Autodesk Inventor part; units mm, degrees
ref_plane "YZ Plane" through (0, 0, 0) normal (1, 0, 0) x (0, 1, 0)
ref_plane "XZ Plane" through (0, 0, 0) normal (0, 1, 0) x (-1, 0, 0)
ref_plane "XY Plane" through (0, 0, 0) normal (0, 0, 1) x (1, 0, 0)
sketch "Sketch1" plane through (0, 0, 0) normal (0, 1, 0) x (-1, 0, 0)
  circle A0 centre (0, 0) radius 19.4
  line L0 (0, 0) -> (0, -10.9961) construction
  circle A1 centre (0, -45) radius 19.4
  circle A2 centre (45, 22.5) radius 19.4
  circle A3 centre (45, -22.5) radius 19.4
  circle A4 centre (45, -67.5) radius 19.4
  line L1 (-27.5, -92.5) -> (72.5, -92.5)
  line L2 (72.5, -92.5) -> (72.5, 47.5)
  line L3 (72.5, 47.5) -> (-27.5, 47.5)
  line L4 (-27.5, 47.5) -> (-27.5, -92.5)
  line L5 (-27.5, -92.5) -> (72.5, 47.5) construction
  line L6 (72.5, -92.5) -> (-27.5, 47.5) construction
  point P0 (22.5, -22.5)
  dimension "d0" = 38.8
  dimension "d3" = 45
  dimension "d8" = 38.8
  dimension "d9" = 45
  dimension "d10" = 22.5
  dimension "d13" = 45
  dimension "d18" = 22.5
  dimension "d19" = 50
  dimension "d20" = 70
  dimension "d21" = 22.5
extrude "Extrusion1" add sketch "Sketch1" along normal blind 10
extrude "Extrusion2" add sketch "Sketch1" against normal blind 3 contours A0 | A1 | A2 | A3 | A4 | L4 L3 L2 L1
sketch "Sketch3" plane through (0, 10, 0) normal (0, 1, 0) x (1, 0, 0)
  line L0 (24.5, 89.5) -> (19.5, 89.5)
  line L1 (19.5, 89.5) -> (19.5, 84.5)
  line L2 (19.5, 84.5) -> (24.5, 84.5)
  line L3 (24.5, 84.5) -> (24.5, 89.5)
  line L4 (24.5, -39.5) -> (19.5, -39.5)
  line L5 (19.5, -39.5) -> (19.5, -44.5)
  line L6 (19.5, -44.5) -> (24.5, -44.5)
  line L7 (24.5, -44.5) -> (24.5, -39.5)
  line L8 (-64.5, -44.5) -> (-69.5, -44.5)
  line L9 (-69.5, -44.5) -> (-69.5, -39.5)
  line L10 (-69.5, -39.5) -> (-64.5, -39.5)
  line L11 (-64.5, -39.5) -> (-64.5, -44.5)
  line L12 (-64.5, 89.5) -> (-69.5, 89.5)
  line L13 (-69.5, 89.5) -> (-69.5, 84.5)
  line L14 (-69.5, 84.5) -> (-64.5, 84.5)
  line L15 (-64.5, 84.5) -> (-64.5, 89.5)
  line L16 (27.5, -47.5) -> (27.5, 92.5)
  line L17 (27.5, 92.5) -> (-72.5, 92.5)
  line L18 (-72.5, -47.5) -> (27.5, -47.5)
  line L19 (-72.5, 92.5) -> (-72.5, -47.5)
  point P0 (0, 0)
  dimension "d26" = 5
  dimension "d27" = 3
  dimension "d28" = 3
  dimension "d29" = 5
  dimension "d30" = 3
  dimension "d31" = 3
  dimension "d32" = 5
  dimension "d33" = 3
  dimension "d34" = 5
extrude "Extrusion3" cut sketch "Sketch3" against normal blind 2 contours L3 L2 L1 L0 | L7 L6 L5 L4 | L8 L9 L10 L11 | L15 L14 L13 L12
equation "\"d0\" = bottleDiameter"
equation "\"d3\" = bottleDistance"
equation "\"d8\" = bottleDiameter"
equation "\"d13\" = bottleDistance"
equation "\"capDiameter\" = 29.5"
equation "\"bottleLen\" = 81.3"
equation "\"bottleDiameter\" = 38.8"
equation "\"tubeInsideDiameter\" = 2"
equation "\"tubeOutsideDiameter\" = 5.4"
equation "\"tick\" = 2"
equation "\"connectorDiameter\" = 35"
equation "\"connectorInsideDiameter\" = tubeInsideDiameter - tick"
equation "\"connectorTubeDepth\" = 18.5"
equation "\"tubeFlapDepth\" = 3"
equation "\"tubeFlapAngle\" = 15deg"
equation "\"minTick\" = 0.25"
equation "\"tubeLinkTick\" = 2"
equation "\"tubeTolerance\" = 0.3"
equation "\"tickHolder\" = 1"
equation "\"bottleDistance\" = 45"
properties part number "trayB"
CAD build for the part. Positions are in the model's coordinates, mm. A direction names the side the tool comes from. Coordinates: 2 decimals unless noted, no trailing zeros. Write each loop counter-clockwise with the first axis right and the second up, starting at its lowest first coordinate (ties: lowest second). Pieces come first, ordered by that corner, then holes.
(1) Cut at A-A, the plane y = 2. List the corners of the cut face in (x, z).
(2) Flat gauge pins, fed straight in: pin 1 (3 mm diameter, centred on x = 8, z = -13.5, fed in from +Y); pin 2 (4 mm diameter, centred on x = 22, z = 41, fed in from +Y); pin 3 (4 mm diameter, centred on x = -67, z = 42, fed in from +Y). Where does each tip first touch, or does it go through?
(3) Two-plate mould, pull along X, no slides. Class faces 3 (the face through (-11, 10, -22)), 4 (the face through (-72.5, 3, -23)), 5 (the face through (0, 0, -45)): +X half, -X half, draft (parallel to the pull), parting line (faces both ways), or undercut.
(4) Cut at C-C, the plane z = -22.5. List the corners of the cut face in (x, y).
(5) Drill centre lines: probe 1 along Z at (x, y) = (-45, 3.25); probe 2 along Z at (x, y) = (0, 7.75); probe 3 along Z at (x, y) = (14, 6.5). Where is each one in solid material? Low to high.
(6) Cut at D-D, the plane z = 17. List the corners of the cut face in (x, y).
(7) 3-axis set-ups, long thin cutter, end or side, ignore diameter. For faces 1 (the face through (-22, 3, -92.5)), 2 (the face through (22, 8, -87)): which of +Z, -Z, +X, -X, +Y, -Y reach the whole face in a straight line?
(8) Cut at B-B, the plane x = -32. List the corners of the cut face in (y, z).
Geometry says:
1. outline: (-72.5, -92.5) - (27.5, -92.5) - (27.5, 47.5) - (-72.5, 47.5) - close; hole circle Ø38.8 at (-45, -67.5); hole circle Ø38.8 at (-45, -22.5); hole circle Ø38.8 at (-45, 22.5); hole circle Ø38.8 at (0, -45); hole circle Ø38.8 at (0, 0)
2. pin 1: stops at y = 0
2. pin 2: stops at y = 10
2. pin 3: stops at y = 8
3. face 3: draft
3. face 4: -X half
3. face 5: undercut
4. outline: (-72.5, -3) - (27.5, -3) - (27.5, 10) - (-25.6, 10) - (-25.6, 0) - (-64.4, 0) - (-64.4, 10) - (-72.5, 10) - close
5. probe 1: z = -92.5 to -86.9, -48.1 to -41.9, -3.1 to 3.1, 41.9 to 47.5
5. probe 2: z = -92.5 to -64.4, -25.6 to -19.4, 19.4 to 47.5
5. probe 3: z = -92.5 to -58.43, -31.57 to -13.43, 13.43 to 47.5
6. outline: (-72.5, -3) - (27.5, -3) - (27.5, 10) - (9.35, 10) - (9.35, 0) - (-9.35, 0) - (-9.35, 10) - (-26.4, 10) - (-26.4, 0) - (-63.6, 0) - (-63.6, 10) - (-72.5, 10) - close
7. face 1: -Z, +X, -X, +Y, -Y
7. face 2: +Y
8. outline: (-3, -92.5) - (10, -92.5) - (10, -81.9) - (0, -81.9) - (0, -53.1) - (10, -53.1) - (10, -36.9) - (0, -36.9) - (0, -8.1) - (10, -8.1) - (10, 8.1) - (0, 8.1) - (0, 36.9) - (10, 36.9) - (10, 47.5) - (-3, 47.5) - close
